Autodesk Inventor part; units mm, degrees
ref_plane "YZ Plane" through (0, 0, 0) normal (1, 0, 0) x (0, 1, 0)
ref_plane "XZ Plane" through (0, 0, 0) normal (0, 1, 0) x (-1, 0, 0)
ref_plane "XY Plane" through (0, 0, 0) normal (0, 0, 1) x (1, 0, 0)
sketch "Sketch1" plane through (0, 0, 0) normal (0, 1, 0) x (-1, 0, 0)
  line L0 (-17.9221, -16.5) -> (-498.4221, -16.5)
  line L1 (-518.4221, 3.5) -> (-518.4221, 130)
  line L2 (-498.4221, 150) -> (251.5779, 150)
  line L3 (271.5779, 130) -> (271.5779, 30)
  line L4 (-18.4221, -12) -> (-498.4221, -12)
  line L5 (-513.9221, 3.5) -> (-513.9221, 130)
  line L6 (-498.4221, 145.5) -> (251.5779, 145.5)
  line L7 (267.0779, 130) -> (267.0779, 30)
  line L8 (251.5779, 14.5) -> (-488.9221, 14.5)
  line L9 (-504.4221, 30) -> (-504.4221, 120.5)
  line L10 (251.5779, 10) -> (-488.9221, 10)
  line L11 (-508.9221, 30) -> (-508.9221, 120.5)
  line L12 (-488.9221, 136) -> (242.0779, 136)
  line L13 (-488.9221, 140.5) -> (242.0779, 140.5)
  line L14 (257.5779, 120.5) -> (257.5779, 56.5)
  line L15 (242.0779, 41) -> (-479.4221, 41)
  line L16 (262.0779, 120.5) -> (262.0779, 56.5)
  line L17 (242.0779, 36.5) -> (-479.4221, 36.5)
  line L18 (-494.9221, 56.5) -> (-494.9221, 111)
  line L19 (-479.4221, 126.5) -> (232.5779, 126.5)
  line L20 (248.0779, 111) -> (248.0779, 83)
  line L21 (232.5779, 67.5) -> (-488.9221, 67.5)
  line L22 (-499.4221, 56.5) -> (-499.4221, 111)
  line L23 (-479.4221, 131) -> (232.5779, 131)
  line L24 (252.5779, 111) -> (252.5779, 83)
  line L25 (232.5779, 63) -> (-488.9221, 63)
  line L26 (-122.9221, 150) -> (-122.9221, -150) construction
  line L27 (-18.9221, -12) -> (251.5779, -12)
  line L28 (271.5779, -32) -> (271.5779, -129.5)
  line L29 (251.5779, -149.5) -> (-498.4221, -149.5)
  line L30 (-518.4221, -129.5) -> (-518.4221, -58.5)
  line L31 (-18.9221, -16.5) -> (251.5779, -16.5)
  line L32 (267.0779, -32) -> (267.0779, -129.5)
  line L33 (251.5779, -145) -> (-498.4221, -145)
  line L34 (-498.4221, -38.5) -> (242.0779, -38.5)
  line L35 (262.0779, -58.5) -> (262.0779, -120)
  line L36 (242.0779, -140) -> (-488.9221, -140)
  line L37 (-513.9221, -129.5) -> (-513.9221, -58.5)
  line L38 (-498.4221, -43) -> (242.0779, -43)
  line L39 (257.5779, -58.5) -> (257.5779, -120)
  line L40 (242.0779, -135.5) -> (-488.9221, -135.5)
  line L41 (-504.4221, -120) -> (-504.4221, -85)
  line L42 (-508.9221, -120) -> (-508.9221, -85)
  line L43 (-488.9221, -65) -> (232.5779, -65)
  line L44 (252.5779, -85) -> (252.5779, -110.5)
  line L45 (-488.9221, -69.5) -> (232.5779, -69.5)
  line L46 (248.0779, -85) -> (248.0779, -110.5)
  line L47 (232.5779, -126) -> (-488.9221, -126)
  line L48 (232.5779, -130.5) -> (-488.9221, -130.5)
  line L49 (276.5779, 200.5) -> (276.5779, -199.5)
  line L50 (276.5779, -199.5) -> (-523.4221, -199.5)
  line L51 (-523.4221, -199.5) -> (-523.4221, 200)
  line L52 (-523.4221, 200) -> (276.5779, 200)
  line L53 (276.5779, 200) -> (276.5779, -199.5)
  arc A0 (251.5779, -149.5) -> (271.5779, -129.5) centre (251.5779, -129.5) ccw
  arc A1 (251.5779, -145) -> (267.0779, -129.5) centre (251.5779, -129.5) ccw
  arc A2 (242.0779, -135.5) -> (257.5779, -120) centre (242.0779, -120) ccw
  arc A3 (242.0779, -140) -> (262.0779, -120) centre (242.0779, -120) ccw
  arc A4 (232.5779, -130.5) -> (252.5779, -110.5) centre (232.5779, -110.5) ccw
  arc A5 (232.5779, -126) -> (248.0779, -110.5) centre (232.5779, -110.5) ccw
  arc A6 (248.0779, -85) -> (232.5779, -69.5) centre (232.5779, -85) ccw
  arc A7 (252.5779, -85) -> (232.5779, -65) centre (232.5779, -85) ccw
  line L54 (266.0656, -58.5) -> (242.0779, -58.5) construction
  line L55 (242.0779, -58.5) -> (242.0779, -27) construction
  arc A8 (257.5779, -58.5) -> (242.0779, -43) centre (242.0779, -58.5) ccw
  arc A9 (262.0779, -58.5) -> (242.0779, -38.5) centre (242.0779, -58.5) ccw
  line L56 (251.5779, -3.7302) -> (251.5779, -32) construction
  line L57 (251.5779, -32) -> (272.6377, -32) construction
  arc A10 (267.0779, -32) -> (251.5779, -16.5) centre (251.5779, -32) ccw
  arc A11 (271.5779, -32) -> (251.5779, -12) centre (251.5779, -32) ccw
  arc A12 (-518.4221, -129.5) -> (-498.4221, -149.5) centre (-498.4221, -129.5) ccw
  arc A13 (-513.9221, -129.5) -> (-498.4221, -145) centre (-498.4221, -129.5) ccw
  arc A14 (-508.9221, -120) -> (-488.9221, -140) centre (-488.9221, -120) ccw
  line L58 (-488.9221, -130.5) -> (-488.9221, -126)
  arc A15 (-504.4221, -120) -> (-488.9221, -135.5) centre (-488.9221, -120) ccw
  arc A16 (-488.9221, -65) -> (-508.9221, -85) centre (-488.9221, -85) ccw
  arc A17 (-488.9221, -69.5) -> (-504.4221, -85) centre (-488.9221, -85) ccw
  arc A18 (-498.4221, -43) -> (-513.9221, -58.5) centre (-498.4221, -58.5) ccw
  arc A19 (-498.4221, -38.5) -> (-518.4221, -58.5) centre (-498.4221, -58.5) ccw
  line L59 (-488.9221, 63) -> (-488.9221, 67.5)
  arc A20 (-518.4221, 3.5) -> (-498.4221, -16.5) centre (-498.4221, 3.5) ccw
  arc A21 (-513.9221, 3.5) -> (-498.4221, -12) centre (-498.4221, 3.5) ccw
  arc A22 (-508.9221, 30) -> (-488.9221, 10) centre (-488.9221, 30) ccw
  arc A23 (-504.4221, 30) -> (-488.9221, 14.5) centre (-488.9221, 30) ccw
  arc A24 (-499.4221, 56.5) -> (-479.4221, 36.5) centre (-479.4221, 56.5) ccw
  arc A25 (-494.9221, 56.5) -> (-479.4221, 41) centre (-479.4221, 56.5) ccw
  arc A26 (-479.4221, 126.5) -> (-494.9221, 111) centre (-479.4221, 111) ccw
  arc A27 (-479.4221, 131) -> (-499.4221, 111) centre (-479.4221, 111) ccw
  arc A28 (-488.9221, 136) -> (-504.4221, 120.5) centre (-488.9221, 120.5) ccw
  arc A29 (-488.9221, 140.5) -> (-508.9221, 120.5) centre (-488.9221, 120.5) ccw
  arc A30 (-498.4221, 145.5) -> (-513.9221, 130) centre (-498.4221, 130) ccw
  arc A31 (-498.4221, 150) -> (-518.4221, 130) centre (-498.4221, 130) ccw
  arc A32 (251.5779, 10) -> (271.5779, 30) centre (251.5779, 30) ccw
  arc A33 (251.5779, 14.5) -> (267.0779, 30) centre (251.5779, 30) ccw
  arc A34 (242.0779, 41) -> (257.5779, 56.5) centre (242.0779, 56.5) ccw
  arc A35 (242.0779, 36.5) -> (262.0779, 56.5) centre (242.0779, 56.5) ccw
  arc A36 (232.5779, 63) -> (252.5779, 83) centre (232.5779, 83) ccw
  arc A37 (232.5779, 67.5) -> (248.0779, 83) centre (232.5779, 83) ccw
  arc A38 (248.0779, 111) -> (232.5779, 126.5) centre (232.5779, 111) ccw
  arc A39 (252.5779, 111) -> (232.5779, 131) centre (232.5779, 111) ccw
  arc A40 (257.5779, 120.5) -> (242.0779, 136) centre (242.0779, 120.5) ccw
  arc A41 (262.0779, 120.5) -> (242.0779, 140.5) centre (242.0779, 120.5) ccw
  arc A42 (267.0779, 130) -> (251.5779, 145.5) centre (251.5779, 130) ccw
  arc A43 (271.5779, 130) -> (251.5779, 150) centre (251.5779, 130) ccw
  circle A44 centre (-493.4221, -169.5) radius 3.25
  circle A45 centre (246.5779, 170) radius 3.25
  point P0 (-228.4221, 0)
  point P1 (276.5779, 200)
  point P2 (257.5779, -126)
  dimension "d2" = 4.5
  dimension "d3" = 4.5
  dimension "d4" = 4.5
  dimension "d5" = 5
  dimension "d6" = 5
  dimension "d7" = 4.5
  dimension "d8" = 4.5
  dimension "d9" = 4.5
  dimension "d10" = 5
  dimension "d11" = 790
  dimension "d12" = 22
  dimension "d13" = 4.5
  dimension "d14" = 4.5
  dimension "d15" = 22
  dimension "d16" = 5
  dimension "d17" = 5
  dimension "d18" = 4.5
  dimension "d19" = 5
  dimension "d20" = 22
  dimension "d21" = 4.5
  dimension "d22" = 4.5
  dimension "d23" = 4.5
  dimension "d30" = 4.5
  dimension "d31" = 4.5
  dimension "d32" = 4.5
  dimension "d34" = 500
  dimension "d35" = 4.5
  dimension "d36" = 4.5
  dimension "d38" = 4.5
  dimension "d39" = 22
  dimension "d40" = 4.5
  dimension "d41" = 5
  dimension "d42" = 4.5
  dimension "d43" = 4.5
  dimension "d44" = 4.5
  dimension "d46" = 22
  dimension "d47" = 5
  dimension "d48" = 4.5
  dimension "d49" = 5
  dimension "d63" = 400
  dimension "d64" = 50
  dimension "d65" = 5
  dimension "d68" = 5
  dimension "d80" = 4.5
  dimension "d81" = 0
  dimension "d103" = 5
  dimension "d126" = 30
  dimension "d127" = 6.5
  dimension "d128" = 30
  dimension "d129" = 6.5
  dimension "d130" = 30
  dimension "d131" = 30
extrude "Extrusion2" add sketch "Sketch1" along normal blind 4.5
equation "\"d6\" = d26"
equation "\"d10\" = d26"
equation "\"d15\" = d28"
equation "\"d16\" = d26"
equation "\"d19\" = d25"
equation "\"d20\" = d28"
equation "\"d41\" = d53"
equation "\"d46\" = d54"
equation "\"d47\" = d53"
equation "\"d49\" = d53"
equation "\"d25\" = 5"
equation "\"d26\" = 5"
equation "\"d28\" = -1.2 * d25 + 0.2 * d29"
equation "\"d51\" = 5"
equation "\"d53\" = 5"
equation "\"d54\" = -1.2 * d51 + 0.2 * d55"
properties part number "wire_holder_lasercutting800"
Build history of the part. All positions in model axes, mm. Give positions to 0.01 mm unless a question says otherwise; leave off trailing zeros.
1) Band-saw the part on A-A on x = -99. State how many separate pieces and enclosed holes the cut face has, then the cut area to 3 significant figures.
Values follow:
separate pieces: 13
enclosed holes: 0
area: 1,550 mm2
2) Two-plate mould, pull along Z, no slides. Class faces 1 (the face through (502.908, 2.218, -134.297)), 2 (the face through (129, 0, 3)): released by +Z, released by -Z, zero draft, split by the parting line, or undercut.
Values follow:
face 1: undercut
face 2: zero draft
3) Probe line 1 along X through (y, z) = (2.45, -103); line 2 along X through (y, z) = (3.1, 138); line 3 along X through (y, z) = (2, -169.5). List the from-to ranges inside material, lowest first.
Values follow:
line 1: x = -276.58 to -271.58, -267.08 to -262.08, -257.58 to -252.58, -248.08 to 504.42, 508.92 to 513.92, 518.42 to 523.42
line 2: x = -276.58 to -269.91, -264.85 to -251.76, 498.6 to 511.7, 516.75 to 523.42
line 3: x = -276.58 to 490.17, 496.67 to 523.42
4) Drop a flat-ended pin along its axis: P1, Ø6, axis at x = -246.58, z = 170, coming from the -Y side. Give the stop position or say it passes through.
Values follow:
P1: passes through
